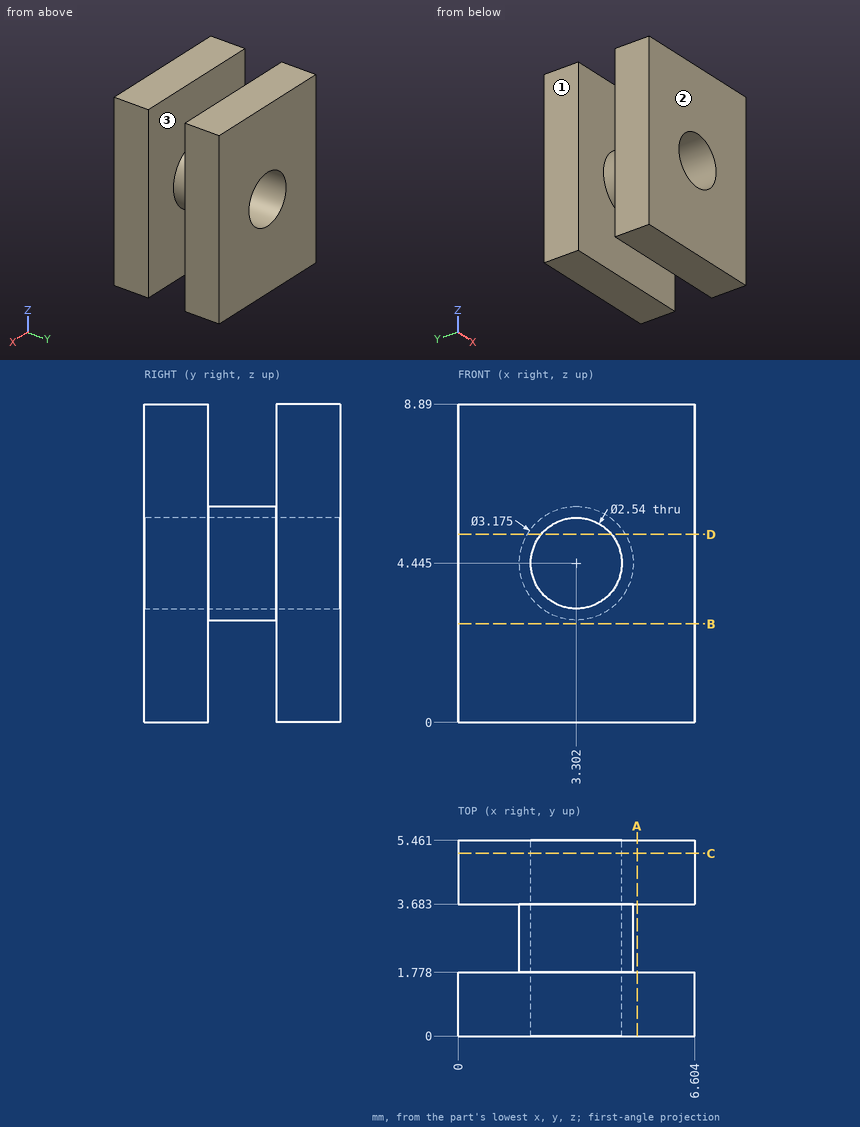
Drawing for the job (mm, zero at the part's lowest x, y, z). Coordinates: 2 decimals unless noted, no trailing zeros. Write each loop counter-clockwise with the first axis right and the second up, starting at its lowest first coordinate (ties: lowest second). Pieces come first, ordered by that corner, then holes. Notation, with made-up numbers: (-18.5, 17) - (-9.5, 17) arc R13 ccw to (-9.5, 28) - close; hole circle Ø4 at (-21.5, -2). An arc over 180 degrees is marked (long way). Write each question's results on one line, items separated by ' | '. Start each with the question number.
1) Mould opens along Y. For the marked faces 1, 2 and 3 say: pulls with the +Y half, pulls with the -Y half, needs draft (parallel to the pull), parting line crosses it, or undercut.
2) Cut at B-B (z = 2.75). Write the cut outline in (x, y), then the cut area to 3 significant figures.
3) Probe line 1 along Y through (x, z) = (1, 2.25); line 2 along X through (y, z) = (2.85, 5.5); line 3 along Z through (x, y) = (3, 0.9). List the from-to ranges inside material, lowest first. Write a range as from..to.
4) Cut at C-C (y = 5.1). Write the cut outline in (x, z) (3 decimals).
5) Cut at D-D (z = 5.25). Write the cut outline in (x, y), then the cut area to 3 significant figures.
6) Cut at A-A (x = 5). Write the cut outline in (y, z), then the cut area to 3 significant figures.
Returned:
1) face 1: needs draft | face 2: pulls with the -Y half | face 3: undercut
2) outline: (0, 0) - (6.6, 0) - (6.6, 1.78) - (0, 1.78) - close; (0, 3.68) - (6.6, 3.68) - (6.6, 5.46) - (0, 5.46) - close | area: 23.5 mm^2
3) line 1: 0..1.78, 3.68..5.46 | line 2: 2.12..2.59, 4.01..4.49 | line 3: 0..3.21, 5.68..8.89
4) outline: (0, 0) - (6.604, 0) - (6.604, 8.89) - (0, 8.89) - close; hole circle Ø2.54 at (3.302, 4.445)
5) outline: (0, 0) - (2.32, 0) - (2.32, 5.46) - (0, 5.46) - (0, 3.68) - (1.93, 3.68) - (1.93, 1.78) - (0, 1.78) - close; (4.28, 0) - (6.6, 0) - (6.6, 1.78) - (4.67, 1.78) - (4.67, 3.68) - (6.6, 3.68) - (6.6, 5.46) - (4.28, 5.46) - close | area: 18.0 mm^2
6) outline: (0, 0) - (1.78, 0) - (1.78, 8.89) - (0, 8.89) - close; (3.68, 0) - (5.46, 0) - (5.46, 8.89) - (3.68, 8.89) - close | area: 31.6 mm^2
